```python
from build123d import *

# Parameters (mm, degrees)
SKETCH1_R           = 7.45
BOSS_EXTRUDE1_DEPTH = 60
SKETCH2_W           = 20
SKETCH2_H           = 20
BOSS_EXTRUDE2_DEPTH = 20
SKETCH3_R           = 7.45
CUT_EXTRUDE1_DEPTH  = 86.893170968


with BuildPart() as part:
    # Sketch1 → Boss-Extrude1 (new body)
    with BuildSketch(Plane.XY):
        with Locations((18.997949105, 14.034076201)):
            Circle(SKETCH1_R)
    extrude(amount=BOSS_EXTRUDE1_DEPTH)

    # Sketch2 → Boss-Extrude2 (add)
    with BuildSketch(Plane.XY.offset(60)):
        with Locations((18.997949105, 14.034076201)):
            Rectangle(SKETCH2_W, SKETCH2_H)
    extrude(amount=BOSS_EXTRUDE2_DEPTH)

    # Sketch3 → Cut-Extrude1 (cut, through all)
    with BuildSketch(Plane(origin=(28.997949105, 0, 0), x_dir=(0, 0, -1), z_dir=(1, 0, 0))):
        with Locations((-70, 14.034076201)):
            Circle(SKETCH3_R)
    extrude(amount=-CUT_EXTRUDE1_DEPTH, mode=Mode.SUBTRACT)


solid = part.part
```
Read the model definition and answer for the solid it produces. Units are mm, in the model's axes. Coordinates: 2 decimals unless noted, no trailing zeros. Write each loop counter-clockwise with the first axis right and the second up, starting at its lowest first coordinate (ties: lowest second). Pieces come first, ordered by that corner, then holes. Notation, with made-up numbers: (3, -21.5) -> (43, -21.5) arc R17 cw to (43, 0.5) -> close; hole circle Ø2 at (-39, -9.5). An arc over 180 degrees is marked (long way). Answer as a JSON object with one key per item and string values.
Q1. Determine the mould class of faces 1 (the flat face through (19, 14, 80)), 2 (the cylindrical face through (13.086, 9.501, 29.58)), 3 (the cylindrical face through (19.138, 14.362, 77.443)), 4 (the flat face through (23, 21, 60)) for opening direction Z: pulls with the +Z half, pulls with the -Z half, needs draft (parallel to the pull), parting line crosses it, or undercut.
The answers:
{"face 1": "pulls with the +Z half", "face 2": "needs draft", "face 3": "undercut", "face 4": "pulls with the -Z half"}
Q2. The part is cut by section C-C on x = 15.5. Give the vertices of the cut face in (y, z).
The answers:
{"outline": "(4.03, 60) -> (7.46, 60) -> (7.46, 0) -> (20.61, 0) -> (20.61, 60) -> (24.03, 60) -> (24.03, 80) -> (4.03, 80) -> close; hole circle Ø14.9 at (14.03, 70)"}
Q3. The part is cut by section A-A on z = 70. Give the vertices of the cut face in (x, y).
The answers:
{"outline": "(9, 4.03) -> (29, 4.03) -> (29, 6.58) -> (9, 6.58) -> close; (9, 21.48) -> (29, 21.48) -> (29, 24.03) -> (9, 24.03) -> close"}
Q4. The part is cut by section D-D on y = 14.75. Give the vertices of the cut face in (x, z).
The answers:
{"outline": "(9, 60) -> (11.58, 60) -> (11.58, 0) -> (26.41, 0) -> (26.41, 60) -> (29, 60) -> (29, 62.58) -> (9, 62.58) -> close; (9, 77.42) -> (29, 77.42) -> (29, 80) -> (9, 80) -> close"}
Q5. The part is cut by section B-B on y = 9.5. Give the vertices of the cut face in (x, z), then the cut area to 3 significant figures.
The answers:
{"outline": "(9, 60) -> (13.09, 60) -> (13.09, 0) -> (24.91, 0) -> (24.91, 60) -> (29, 60) -> (29, 64.09) -> (9, 64.09) -> close; (9, 75.91) -> (29, 75.91) -> (29, 80) -> (9, 80) -> close", "area": "873 mm2"}
Q6. Consider line 1 (Z direction, x = 15.25, y = 14.5); line 2 (Y direction, x = 18, z = 70); line 3 (Z direction, x = 17.75, y = 22.25). Determine where each line is inside the solid, lowest interval first. Write a range as [from, to].
The answers:
{"line 1": "z = [0, 62.56], [77.44, 80]", "line 2": "y = [4.03, 6.58], [21.48, 24.03]", "line 3": "z = [60, 80]"}
Q7. Flat-ended cylindrical pins translate along their axes: pin 1 Ø3 at (y, z) = (20.5, 34.5) entering from -X; pin 2 Ø12 at (x, z) = (19, 28.5) entering from +Y; pin 3 Ø4 at (y, z) = (18, 47.5) entering from -X. Find the tip coordinate at first contact, or state that the pin passes through.
The answers:
{"pin 1": "stops at x = 13.44", "pin 2": "stops at y = 21.48", "pin 3": "stops at x = 11.81"}
